Can you work these out from the model? Positions are in its coordinate system, mm. A direction names the side the tool comes from. Coordinates: 2 decimals unless noted, no trailing zeros. Write each loop counter-clockwise with the first axis right and the second up, starting at its lowest first coordinate (ties: lowest second). Pieces come first, ordered by that corner, then holes. Notation, with made-up numbers: (32.25, 35) - (87.25, 35) arc R19 cw to (87.25, 65) - close; hole circle Ø5 at (77, 56.25). An arc over 180 degrees is marked (long way). Use one line per item in the form item = value. Start each with the question number.
(1) For pin 1 Ø1.7 at (y, z) = (-14, 22) entering from +X; pin 2 Ø6 at (x, z) = (59, 30.5) entering from +Y; pin 3 Ø1.5 at (x, z) = (62, 26.5) entering from +Y, each with a flat end and sliding along its axis, tell me the tip position at first contact or that it passes through.
(2) If we section it at C-C on y = -34: Please give me the cut outline in (x, z) (3 decimals), then the cut area to 3 significant figures.
(3) If I drill on probe 1 along X at (y, z) = (-22, 21); probe 2 along Y at (x, z) = (60.5, 28); probe 3 along Y at (x, z) = (64.5, 27), over which ranges is the centre line in solid material (lowest first)? Write a range as from..to.
(4) Thinking about a two-plate mould opening in X: for faces 5 (the face through (51.54, -5.73, 17.2)), 6 (the face through (67.502, -29.246, 27.143)), 7 (the face through (41.23, -9.05, 18.78)), which applies, pulls with the +X half, pulls with the -X half, needs draft (parallel to the pull), parting line crosses it, or undercut?
(5) On a 3-axis mill with a long thin cutter (end or side, diameter ignored), from which of +Z, -Z, +X, -X, +Y, -Y can I reach the whole of each face in a straight line? I mean faces 1 (the face through (62.6, -15.24, 18.1)), 2 (the face through (63.037, -24, 20)), 3 (the face through (66, -19, 28.575)), 4 (the face through (47.59, -12.89, 13.74)). Say none if no direction works.
(6) If we section it at A-A on z = 33.5: Please give me the cut outline in (x, y).
(7) If we section it at B-B on x = 65.5: Give the number of separate pieces and of enclosed holes in the cut face, then the cut area to 3 significant figures.
```python
from build123d import *

# Parameters (mm, degrees)
F0_W      = 38.1
F0_H      = 38.1
F1_DEPTH  = 38.1
F5_W      = 38.1
F5_H      = 38.1
F6_DEPTH  = 38.1
F1_FACE_W = 38.1
F1_FACE_H = 38.1
F8_DEPTH  = 38.1
F9_DEPTH  = 38.1
F11_DEPTH = 38.1
F13_W     = 28.973644
F13_H     = 7.62
F13_W_2   = 31.493082
F14_DEPTH = 38.1


with BuildPart() as f1:
    # F0 (on Front) → F1 (new body)
    with BuildSketch(Plane.XZ):
        with Locations((19.05, 19.05)):
            Rectangle(F0_W, F0_H)
    extrude(amount=F1_DEPTH)

    # F5 (on offset) → F6 (join)
    with BuildSketch(Plane.YZ.offset(38.1)):
        with Locations((-19.05, 19.05)):
            Rectangle(F5_W, F5_H)
    extrude(amount=F6_DEPTH)

    # F1_face (on face) → F8 (cut)
    with BuildSketch(Plane(origin=(0, -19.05, 19.05), x_dir=(0, -1, 0), z_dir=(-1, 0, 0))):
        Rectangle(F1_FACE_W, F1_FACE_H)
    extrude(amount=-F8_DEPTH, mode=Mode.SUBTRACT)

    # F7 (on face) → F9 (cut)
    with BuildSketch(Plane.YZ.offset(76.2)):
        Polygon((-6.35, 38.1), (-31.75, 38.1), (-26.67, 15.875), (-21.59, 28.575), (-16.51, 28.575), (-11.43, 15.875), align=None)
        Polygon((-19.05, 15.875), (-25.4, 0), (-12.7, 0), align=None)
        Polygon((0, 0), (0, 38.1), (-6.35, 0), align=None)
        Polygon((-31.75, 0), (-38.1, 38.1), (-38.1, 0), align=None)
    extrude(amount=-F9_DEPTH, mode=Mode.SUBTRACT)

    # F10 (on offset) → F11 (cut)
    with BuildSketch(Plane.XZ.offset(38.1)):
        Polygon((63.5, 38.1), (50.8, 38.1), (57.15, 22.225), align=None)
        Polygon((49.53, 22.225), (44.45, 0), (69.85, 0), (64.77, 22.225), (59.69, 9.525), (54.61, 9.525), align=None)
        Polygon((69.85, 38.1), (76.2, 0), (76.2, 38.1), align=None)
        Polygon((38.1, 38.1), (38.1, 0), (44.45, 38.1), align=None)
    extrude(amount=-F11_DEPTH, mode=Mode.SUBTRACT)

    # F13 (on face) → F14 (cut)
    with BuildSketch(Plane.XY.offset(38.1)):
        with Locations((64.823925, -11.43)):
            Rectangle(F13_W, F13_H)
        with Locations((47.290562, -26.67)):
            Rectangle(F13_W_2, F13_H)
    extrude(amount=-F14_DEPTH, mode=Mode.SUBTRACT)


solid = f1.part
```
Reported:
q1.pin_1 = 50.34
q1.pin_2 = -0.94
q1.pin_3 = -1.81
q2.outline = (40.35, 13.5) - (47.536, 13.5) - (49.53, 22.225) - (53.02, 13.5) - (61.28, 13.5) - (64.77, 22.225) - (66.764, 13.5) - (73.95, 13.5) - (69.85, 38.1) - (63.5, 38.1) - (57.15, 22.225) - (50.8, 38.1) - (44.45, 38.1) - close
q2.area = 577 mm2
q3.probe_1 = 41.6..49.25, 50.02..64.28, 65.05..72.7
q3.probe_2 = -36.42..-30.48, -21.82..-16.28, -7.62..-1.68
q3.probe_3 = -36.25..-29.21, -22.22..-15.88, -7.62..-1.85
q4.face_5 = undercut
q4.face_6 = needs draft
q4.face_7 = pulls with the -X half
q5.face_1 = +Z, -Z, +X
q5.face_2 = +Z, -Z, -X
q5.face_3 = +Z, +X, -X
q5.face_4 = -Z, +Y, -Y
q6.outline = (43.68, -37.33) - (52.64, -37.33) - (52.64, -30.7) - (43.68, -30.7) - close; (43.68, -7.4) - (52.64, -7.4) - (52.64, -0.77) - (43.68, -0.77) - close; (61.66, -37.33) - (70.62, -37.33) - (70.62, -30.7) - (61.66, -30.7) - close; (61.66, -7.4) - (70.62, -7.4) - (70.62, -0.77) - (61.66, -0.77) - close
q7.separate_pieces = 3
q7.enclosed_holes = 0
q7.area = 321 mm2
